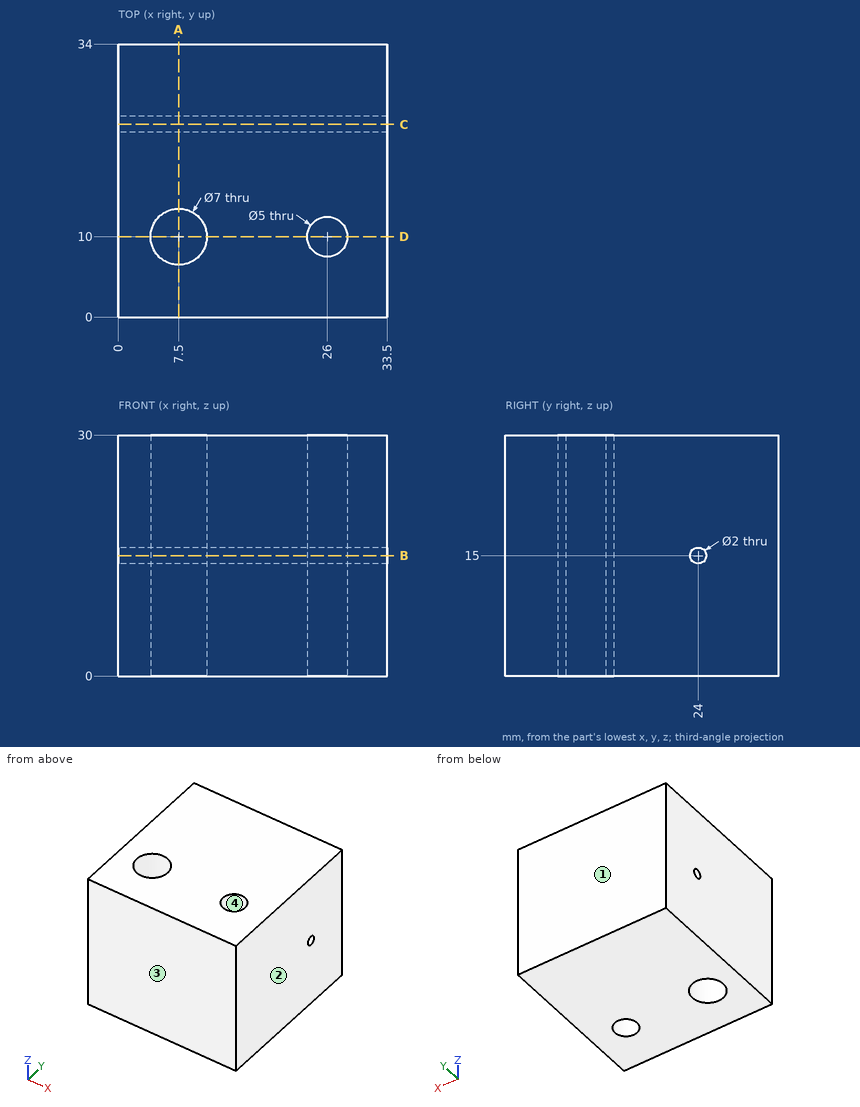
Here's the drawing with two shaded views (mm, measured from the low corner). I have some questions. Round coordinates to 2 decimals unless told otherwise and drop trailing zeros. Write each loop counter-clockwise with the first axis right and the second up, starting at its lowest first coordinate (ties: lowest second). Pieces come first, ordered by that corner, then holes. Notation, with made-up numbers: M -8.5,-24 L 35.5,-24 A5 cw 35.5,-20 Z; hole C 52,-37 d11. An arc over 180 degrees is marked long. Use CSV: the item, a comma, the result in double quotes.
(1) Imagine slicing it at A-A (x = 7.5). Write out the boundary of the cut face in (y, z), plus the area to 3 significant figures.
Check values:
outline,"M 0,0 L 6.5,0 L 6.5,30 L 0,30 Z; M 13.5,0 L 34,0 L 34,30 L 13.5,30 Z; hole C 24,15 d2"
area,"807 mm^2"
(2) Imagine slicing it at B-B (z = 15). Write out the boundary of the cut face in (x, y), plus the area to 3 significant figures.
Check values:
outline,"M 0,0 L 33.5,0 L 33.5,23 L 0,23 Z; M 0,25 L 33.5,25 L 33.5,34 L 0,34 Z; hole C 7.5,10 d7; hole C 26,10 d5"
area,"1,010 mm^2"
(3) We'd pull the mould along Y, two halves only. Please class the marked faces 1, 2, 3 and 4: +Y half, -Y half, draft (parallel to the pull), parting line (faces both ways), or undercut.
Check values:
face 1,"+Y half"
face 2,"draft"
face 3,"-Y half"
face 4,"undercut"
(4) I need wall thicknesses on line 1 along Z through (x, y) = (31, 24); line 2 along X through (y, z) = (8.5, 4.5); line 3 along Y through (x, z) = (7.5, 19.5). Which ranges of each line are inside material? Lowest first, please.
Check values:
line 1,"0 to 14, 16 to 30"
line 2,"0 to 4.34, 10.66 to 24, 28 to 33.5"
line 3,"0 to 6.5, 13.5 to 34"
(5) I'm going to push a flat-ended pin straight in: pin 1 (5.5 mm diameter, centred on x = 7.5, y = 10, fed in from -Z). Where does the tip first touch, or does it pass through?
Check values:
pin 1,"through"
(6) Imagine slicing it at D-D (y = 10). Write out the boundary of the cut face in (x, z).
Check values:
outline,"M 0,0 L 4,0 L 4,30 L 0,30 Z; M 11,0 L 23.5,0 L 23.5,30 L 11,30 Z; M 28.5,0 L 33.5,0 L 33.5,30 L 28.5,30 Z"
(7) Imagine slicing it at C-C (y = 24). Write out the boundary of the cut face in (x, z), plus the area to 3 significant figures.
Check values:
outline,"M 0,0 L 33.5,0 L 33.5,14 L 0,14 Z; M 0,16 L 33.5,16 L 33.5,30 L 0,30 Z"
area,"938 mm^2"
